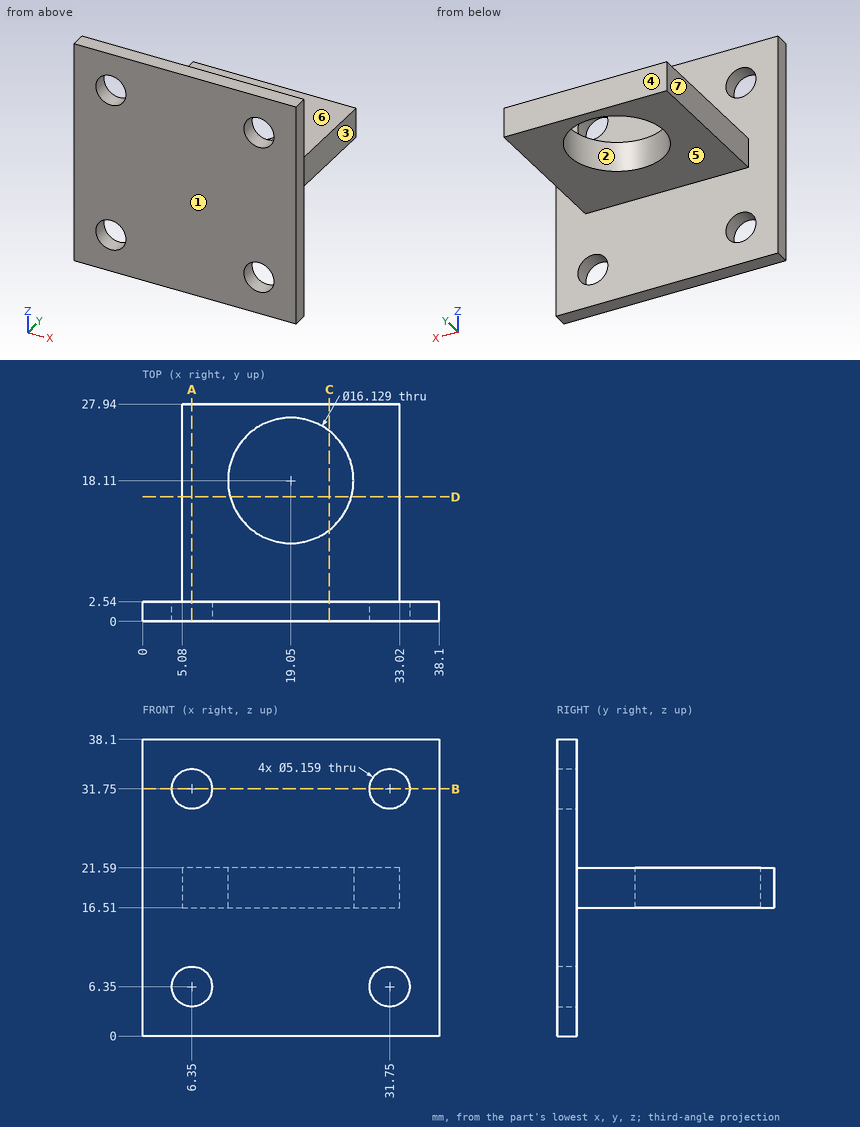
Part print with two shaded views. Sizes in mm from the minimum x, y, z corner. A direction names the side the tool comes from. Round coordinates to 2 decimals unless told otherwise and drop trailing zeros. Write each loop counter-clockwise with the first axis right and the second up, starting at its lowest first coordinate (ties: lowest second). Pieces come first, ordered by that corner, then holes. Notation, with made-up numbers: (71, 26) - (114, 26) arc R15 ccw to (114, 39) - close; hole circle Ø10 at (46.5, 21.5). An arc over 180 degrees is marked (long way). Use CSV: the item, a comma, the result in double quotes.
Item 1: Slice it at A-A, the plane x = 6.35. Write the cut outline in (y, z).
Results list:
outline,"(0, 0) - (2.54, 0) - (2.54, 3.77) - (0, 3.77) - close; (0, 8.93) - (2.54, 8.93) - (2.54, 16.51) - (27.94, 16.51) - (27.94, 21.59) - (2.54, 21.59) - (2.54, 29.17) - (0, 29.17) - close; (0, 34.33) - (2.54, 34.33) - (2.54, 38.1) - (0, 38.1) - close"
Item 2: Slice it at B-B, the plane z = 31.75. Write the cut outline in (x, y).
Results list:
outline,"(0, 0) - (3.77, 0) - (3.77, 2.54) - (0, 2.54) - close; (8.93, 0) - (29.17, 0) - (29.17, 2.54) - (8.93, 2.54) - close; (34.33, 0) - (38.1, 0) - (38.1, 2.54) - (34.33, 2.54) - close"
Item 3: Slice it at D-D, the plane y = 16. Write the cut outline in (x, z).
Results list:
outline,"(5.08, 16.51) - (11.27, 16.51) - (11.27, 21.59) - (5.08, 21.59) - close; (26.83, 16.51) - (33.02, 16.51) - (33.02, 21.59) - (26.83, 21.59) - close"
Item 4: Pull direction Y, two halves, no side cores. Call the marked faces 1, 2, 3 and 4: pulls with the +Y half, pulls with the -Y half, needs draft (parallel to the pull), parting line crosses it, or undercut.
Results list:
face 1,"pulls with the -Y half"
face 2,"undercut"
face 3,"needs draft"
face 4,"pulls with the +Y half"
Item 5: Wall check: L1, parallel to Z at x = 6.35, y = 1.75; L2, parallel to Z at x = 29, y = 26.25; L3, parallel to Y at x = 30, z = 25.5. Give the ranges that are in metal, low to high.
Results list:
L1,"z = 0 to 3.77, 8.93 to 29.17, 34.33 to 38.1"
L2,"z = 16.51 to 21.59"
L3,"y = 0 to 2.54"
Item 6: Slice it at C-C, the plane x = 24. Write the cut outline in (y, z), then the cut area to 3 significant figures.
Results list:
outline,"(0, 0) - (2.54, 0) - (2.54, 16.51) - (11.74, 16.51) - (11.74, 21.59) - (2.54, 21.59) - (2.54, 38.1) - (0, 38.1) - close; (24.48, 16.51) - (27.94, 16.51) - (27.94, 21.59) - (24.48, 21.59) - close"
area,"161 mm²"
Item 7: Flat gauge pins, fed straight in: P1, Ø4, axis at x = 6.35, z = 6.35, coming from the -Y side; P2, Ø7.5, axis at x = 18.5, y = 10, coming from the -Z side; P3, Ø5.5, axis at y = 21, z = 20, coming from the +X side; P4, Ø8.5, axis at x = 31.75, z = 31.75, coming from the +Y side. Where does each tip first touch, or does it go through?
Results list:
P1,"passes through"
P2,"stops at z = 16.51"
P3,"stops at x = 33.02"
P4,"stops at y = 2.54"
Item 8: Tool access for the marked faces 5, 6 and 7: list every direction of +Z, -Z, +X, -X, +Y, -Y with a clear straight run to the whole face (end or side of a thin tool).
Results list:
face 5,"-Z, +X, -X, +Y"
face 6,"+Z, +X, -X, +Y"
face 7,"+Z, -Z, -X, +Y"
